```python
from build123d import *

# Parameters (mm, degrees)
SKETCH_1_W      = 8
SKETCH_1_H      = 8
SKETCH_1_R      = 3
EXTRUDE_1_DEPTH = 60
FILLET_2_R      = 1


with BuildPart() as part:
    # 草图1 → 凸台-拉伸1 (new body)
    # profile 1 of 6: a face of its own
    with BuildSketch(Plane.XY):
        Polygon((10, 11.431478203), (3, 11.431478203), (3, 9.431478203), (5, 9.431478203), (5, 7.431478203), (3, 5.431478203), (4, 5.431478203), (4, 4.431478203), (6, 6.431478203), (8, 6.431478203), (8, 4.431478203), (10, 4.431478203), align=None)
    # profile 2 of 6: a face of its own
    with BuildSketch(Plane.XY):
        Polygon((3, -6.568521797), (3, -8.568521797), (10, -8.568521797), (10, -1.568521797), (8, -1.568521797), (8, -3.568521797), (6, -3.568521797), (4, -1.568521797), (4, -2.568521797), (3, -2.568521797), (5, -4.568521797), (5, -6.568521797), align=None)
    # profile 3 of 6: a face of its own
    with BuildSketch(Plane.XY):
        Polygon((-8, -1.568521797), (-10, -1.568521797), (-10, -8.568521797), (-3, -8.568521797), (-3, -6.568521797), (-5, -6.568521797), (-5, -4.568521797), (-3, -2.568521797), (-4, -2.568521797), (-4, -1.568521797), (-6, -3.568521797), (-8, -3.568521797), align=None)
    # profile 4 of 6: a face of its own
    with BuildSketch(Plane.XY):
        Polygon((-3, 11.431478203), (-10, 11.431478203), (-4, 5.431478203), (-3, 5.431478203), (-5, 7.431478203), (-5, 9.431478203), (-3, 9.431478203), align=None)
    # profile 5 of 6: a face of its own
    with BuildSketch(Plane.XY):
        Polygon((-10, 11.431478203), (-10, 4.431478203), (-8, 4.431478203), (-8, 6.431478203), (-6, 6.431478203), (-4, 4.431478203), (-4, 5.431478203), align=None)
    # profile 6 of 6: a face of its own
    with BuildSketch(Plane.XY):
        with Locations((0, 1.431478203)):
            Rectangle(SKETCH_1_W, SKETCH_1_H)
        with Locations((0, 1.431478203)):
            Circle(SKETCH_1_R, mode=Mode.SUBTRACT)
    extrude(amount=EXTRUDE_1_DEPTH)

    # 圆角2
    fillet_2_edges = [part.edges().sort_by_distance(p)[0] for p in [
        (10, 11.431478203, 30),
        (10, -8.568521797, 30),
        (-10, -8.568521797, 30),
        (-10, 11.431478203, 30),
    ]]
    fillet(fillet_2_edges, radius=FILLET_2_R)


solid = part.part
```
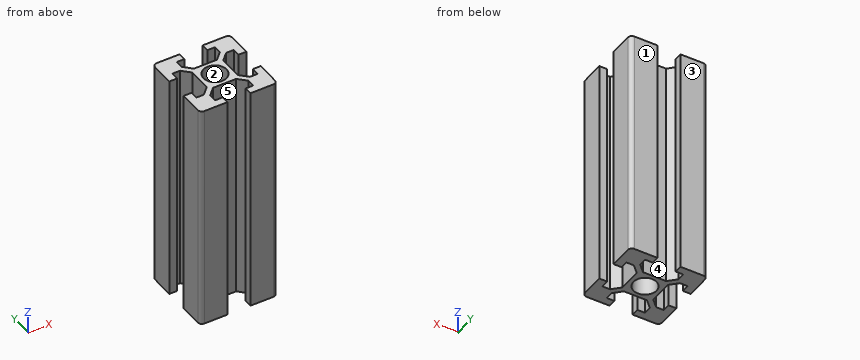
Source: CAD feature listing. Evaluate the final solid. Frame: model axes, mm. Face numbers are marked on the shaded views. A direction names the side the tool comes from. Coordinates: 2 decimals unless noted, no trailing zeros. Order: outer loops, then holes, each group sorted by start corner. A loop starts at its lowest first (then second) coordinate and runs counter-clockwise, first axis right, second up. Notation, with made-up numbers: M 31.5,-17.75 L 79.5,-17.75 A27 cw 79.5,17.25 Z; hole C 0.5,64 d9. An arc over 180 degrees is marked long. Write each question's results on one line, items separated by ' | '. Start each with the question number.
1) Section query B-B (y = 3.25). Return the cut outline in (x, z), plus the area to 3 significant figures.
2) Section query A-A (x = 0). Return the cut outline in (y, z).
3) Draft query along X for the marked faces 1 and 2. Return one class per face: released by +X, released by -X, zero draft, split by the parting line, or undercut.
4) Access query for the marked faces 3, 4 and 5. Directions: +Z, -Z, +X, -X, +Y, -Y. A direction counts if a zero-diameter tool reaches every point of the face in a straight line with its end or side. Return the directions, or none.
5) Line query: line 1 (Y direction, x = 0, z = 47); line 2 (X direction, y = 1.25, z = 43); line 3 (Y direction, x = 9, z = 23). Output: solid intervals per line, ascending. Write a range as from..to.
6) Contact query for flat-ended pins moving along their axis: pin 1 Ø3 at (y, z) = (2.5, 26) entering from +X; pin 2 Ø1 at (y, z) = (3.5, 14) entering from -X; pin 3 Ø3 at (x, z) = (-1, 16) entering from -Y. Output: stop coordinate, or through.
Answers:
1) outline: M -4,0 L -2.39,0 L -2.39,60 L -4,60 Z; M 2.39,0 L 4,0 L 4,60 L 2.39,60 Z | area: 194 mm^2
2) outline: M -2.57,0 L -1.57,0 L -1.57,60 L -2.57,60 Z; M 4.43,0 L 5.43,0 L 5.43,60 L 4.43,60 Z
3) face 1: zero draft | face 2: undercut
4) face 3: +Z, -Z, +X, -X, +Y | face 4: +Z, -Z, +Y | face 5: +Z, -Z, -Y
5) line 1: y = -2.57..-1.57, 4.43..5.43 | line 2: x = -4..-2.99, 2.99..4 | line 3: y = -8.57..-1.57, 4.43..11.43
6) pin 1: stops at x = 4 | pin 2: stops at x = -4 | pin 3: stops at y = -2.57
